For this review, use the dimensioned drawing (mm, ordinates from the lowest corner) and the shaded views. A direction names the side the tool comes from. Give positions to 0.01 mm unless a question says otherwise; leave off trailing zeros. Order: outer loops, then holes, each group sorted by start corner. A loop starts at its lowest first (then second) coordinate and runs counter-clockwise, first axis right, second up. Notation, with made-up numbers: M 19,25.25 L 76,25.25 A26 ccw 76,61.25 Z; hole C 65,20.25 d2. An arc over 180 degrees is marked long. Use CSV: the item, a comma, the result in double quotes. Start each with the question number.
(1) Consider section C-C (x = 12.25). Write out the cut boundary in (y, z).
(2) Consider section B-B (y = 17.5). Write out the cut boundary in (x, z) (1 decimal).
(3) Wall thickness on L1, parallel to Z at x = 11, y = 5.5; L2, parallel to X at y = 14, z = 7.75 (1 decimal); L3, parallel to Y at x = 5.5, z = 2.75: over which ranges is each line inside the solid? List them lowest first. Write a range as from..to.
(4) Consider section D-D (z = 4.75). Write out the cut boundary in (x, y).
(5) Clearance check with flat-ended pins moving along their axes: P1, Ø4, axis at y = 20, z = 11.5, coming from the +X side (1 decimal); P2, Ø2.5, axis at x = 7, y = 17.5, coming from the +Z side; P3, Ø2.5, axis at y = 12, z = 7, coming from the -X side (1 decimal). State where each tip first meets the part, or that it passes through.
(6) Tool access review of the marked faces 1, 2 and 3: name each direction out of +Z, -Z, +X, -X, +Y, -Y from which nothing blocks a thin tool from reaching the whole face with its end or side.
(7) Consider section A-A (z = 1.75). Write out the cut boundary in (x, y), and give its area (3 significant figures).
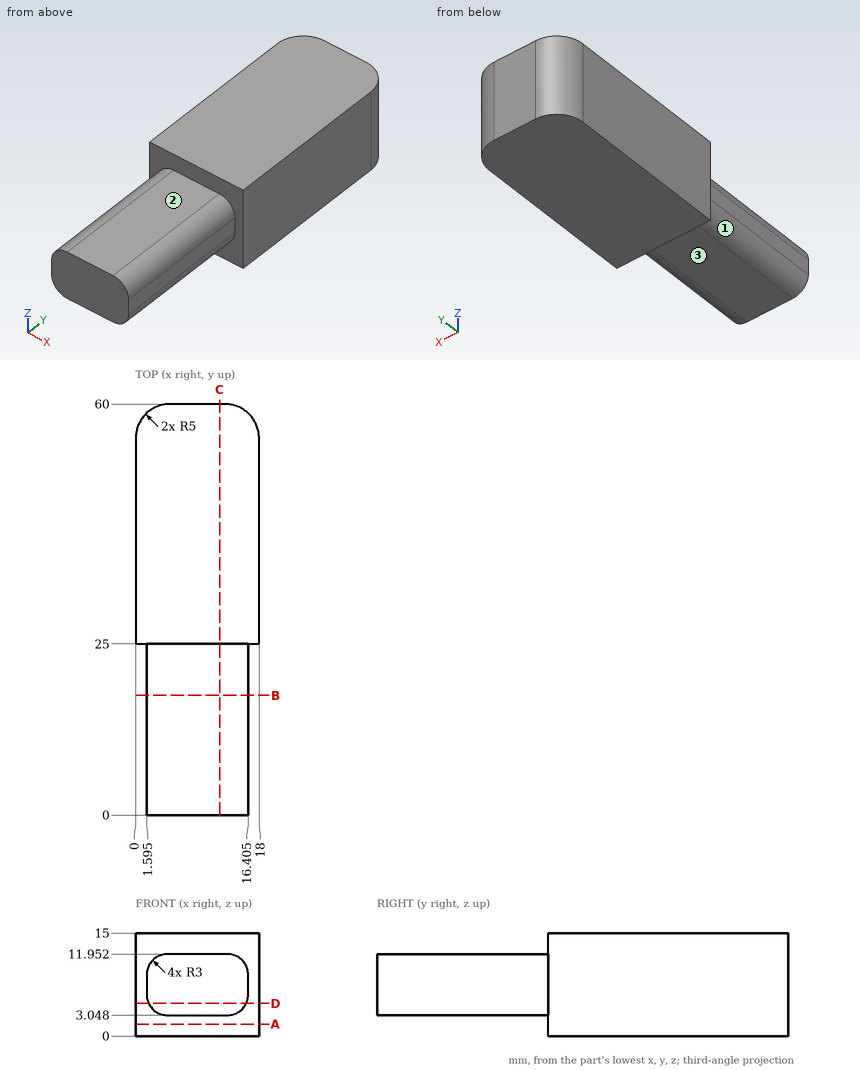
Check result:
1,outline,"M 0,3.05 L 25,3.05 L 25,0 L 60,0 L 60,15 L 25,15 L 25,11.95 L 0,11.95 Z"
2,outline,"M 1.6,6 A3 ccw 4.6,3 L 13.4,3 A3 ccw 16.4,6 L 16.4,9 A3 ccw 13.4,12 L 4.6,12 A3 ccw 1.6,9 Z"
3,L1,"z = 3.05..11.95"
3,L2,"x = 1.6..16.4"
3,L3,"y = 25..60"
4,outline,"M 0,25 L 1.89,25 L 1.89,0 L 16.11,0 L 16.11,25 L 18,25 L 18,55 A5 ccw 13,60 L 5,60 A5 ccw 0,55 Z"
5,P1,"stops at x = 16.4"
5,P2,"stops at z = 11.95"
5,P3,"stops at x = 1.6"
6,face 1,"-Z, -X, -Y"
6,face 2,"+Z, +X, -X, -Y"
6,face 3,"-Z, +X, -X, -Y"
7,outline,"M 0,25 L 18,25 L 18,55 A5 ccw 13,60 L 5,60 A5 ccw 0,55 Z"
7,area,"619 mm^2"
